from build123d import *

# Parameters (mm, degrees)
SKETCH1_R           = 22.225
SKETCH1_R_2         = 17.78
BOSS_EXTRUDE1_DEPTH = 50.8
SKETCH2_R           = 47.625
SKETCH2_R_2         = 22.225
BOSS_EXTRUDE2_DEPTH = 6.35
SKETCH3_R           = 3.175
CUT_EXTRUDE1_DEPTH  = 85.361847123
CHAMFER1_SIZE       = 1.27
BOSS_EXTRUDE3_DEPTH = 1.5875
CIRPATTERN1_COUNT   = 8
CUT_EXTRUDE3_DEPTH  = 85.361847123


with BuildPart() as part:
    # Sketch1 → Boss-Extrude1 (new body)
    with BuildSketch(Plane.XY):
        Circle(SKETCH1_R)
        Circle(SKETCH1_R_2, mode=Mode.SUBTRACT)
    extrude(amount=BOSS_EXTRUDE1_DEPTH)



with BuildPart() as body_2:
    # Sketch2 → Boss-Extrude2 (new body)
    with BuildSketch(Plane.XY.offset(50.8)):
        Circle(SKETCH2_R)
        Circle(SKETCH2_R_2, mode=Mode.SUBTRACT)
    extrude(amount=-BOSS_EXTRUDE2_DEPTH)

    # Sketch3 → Cut-Extrude1 (cut, through all)
    with BuildSketch(Plane.XY.offset(50.8)):
        with Locations((-38.1, 0)):
            Circle(SKETCH3_R)
        with Locations((-26.940768363, 26.940768363)):
            Circle(SKETCH3_R)
        with Locations((0, 38.1)):
            Circle(SKETCH3_R)
        with Locations((26.940768363, 26.940768363)):
            Circle(SKETCH3_R)
        with Locations((38.1, 0)):
            Circle(SKETCH3_R)
        with Locations((26.940768363, -26.940768363)):
            Circle(SKETCH3_R)
        with Locations((0, -38.1)):
            Circle(SKETCH3_R)
        with Locations((-26.940768363, -26.940768363)):
            Circle(SKETCH3_R)
    extrude(amount=-CUT_EXTRUDE1_DEPTH, mode=Mode.SUBTRACT)

    # Chamfer1
    chamfer1_edges = [body_2.edges().sort_by_distance(p)[0] for p in [
        (-47.625, 0, 44.45),
    ]]
    chamfer(chamfer1_edges, length=CHAMFER1_SIZE)


with BuildPart() as part_1:
    add(part.part)

    add(body_2.part)  # Boss-Extrude3 merges body 2
    # Sketch4 → Boss-Extrude3 (add, symmetric)
    with BuildSketch(Plane(origin=(0, 0, 0), x_dir=(0, 0, -1), z_dir=(0.9238795325112865, -0.3826834323650906, 0))):
        Polygon((-44.45, 34.925), (0, 22.225), (0, 21.463), (-44.45, 21.463), align=None)
    boss_extrude3 = extrude(amount=BOSS_EXTRUDE3_DEPTH, both=True)

    # CirPattern1: Boss-Extrude3 ×8 about axis
    cirpattern1_axis = Axis((0, 0, 0), (0, 0, 1))
    for i in range(1, CIRPATTERN1_COUNT):
        add(boss_extrude3.rotate(cirpattern1_axis, i * 360 / CIRPATTERN1_COUNT))

    # Sketch6 → Cut-Extrude3 (cut, through all)
    with BuildSketch(Plane(origin=(0, 0, 0), x_dir=(-1, 0, 0), z_dir=(0, 0, -1))):
        with BuildLine():
            ThreePointArc((-7.572075345, -16.087015726), (-17.372275069, -3.785823414), (-13.579066648, 11.477689183))
            Line((-13.579066648, 11.477689183), (-14.54899998, 12.297524124))
            ThreePointArc((-14.54899998, 12.297524124), (-18.61315186, -4.056239373), (-8.112937869, -17.236088278))
            Line((-8.112937869, -17.236088278), (-7.572075345, -16.087015726))
        make_face()
        with BuildLine():
            ThreePointArc((-10.145726618, 14.601117471), (5.407518283, 16.937743239), (16.729503733, 6.020972085))
            Line((16.729503733, 6.020972085), (17.924468285, 6.45104152))
            ThreePointArc((17.924468285, 6.45104152), (5.793769589, 18.147582041), (-10.870421376, 15.644054433))
            Line((-10.870421376, 15.644054433), (-10.145726618, 14.601117471))
        make_face()
        with BuildLine():
            Line((18.983359245, 1.592033845), (17.717801962, 1.485898255))
            ThreePointArc((17.717801962, 1.485898255), (17.764443685, 0.743599728), (17.78, 0))
            ThreePointArc((17.78, 0), (11.404245451, -13.640805903), (-3.150437085, -17.498661268))
            Line((-3.150437085, -17.498661268), (-3.375468305, -18.748565644))
            ThreePointArc((-3.375468305, -18.748565644), (12.81938227, -14.091342669), (18.983359245, 1.592033845))
        make_face()
    extrude(amount=-CUT_EXTRUDE3_DEPTH, mode=Mode.SUBTRACT)


solid = part_1.part
The listing builds one solid part. Answer for the finished solid, in the listing's coordinates (mm). A direction names the side the tool comes from. Coordinates: 2 decimals unless noted, no trailing zeros. Order: outer loops, then holes, each group sorted by start corner. A loop starts at its lowest first (then second) coordinate and runs counter-clockwise, first axis right, second up. Notation, with made-up numbers: (74, 26) -> (103, 26) arc R28 ccw to (103, 63) -> close; hole circle Ø3 at (47.5, 40.25). An arc over 180 degrees is marked (long way). Answer in a Markdown table with one row per item. Add a question column.
Item 1: Each of these flat-tipped pins is pushed along its axis until it touches: P1, Ø6, axis at y = 29, z = 23, coming from the -X side; P2, Ø1.5, axis at y = 16, z = 19, coming from the -X side; P3, Ø2, axis at y = 11, z = 9, coming from the -X side; P4, Ø5, axis at x = 26.94, y = -26.94, coming from the +Z side (3 decimals). Where does it stop, or does it pass through?
Item 2: Find section A-A (x = 0). Write down the section's boundary in (y, z) (3 decimals), then the cut area to 3 significant figures.
Item 3: Find the intervals of material crossed by L1, parallel to Y at x = 0, z = 46.5 (3 decimals); L2, parallel to Y at x = -29.5, z = 48.5; L3, parallel to Z at x = -4, y = -22, in increasing order. Write a range as from..to.
Item 4: Which of the six approach directions +Z, -Z, +X, -X, +Y, -Y give full straight-line access (tool end or side, diameter ignored) to faces 5 (the face through (22.225, -0.1, 21.914)), 6 (the face through (15.64, -15.79, 21.91)), 7 (the face through (-17.365, 3.818, 25.044)), 8 (the face through (-24.445, -8.407, 31.792))?
Item 5: Determine the mould class of faces 1 (the face through (-18, 5, 0)), 2 (the face through (26.473, -10.99, 22.536)), 3 (the face through (34.93, 0.14, 47.67)), 4 (the face through (15.79, 15.64, 21.91)) for opening direction Y: +Y half, -Y half, draft (parallel to the pull), parting line (faces both ways), or undercut.
Result set:
| question | item | result |
|---|---|---|
| 1 | P1 | stops at x = -12.65 |
| 1 | P2 | stops at x = -16.17 |
| 1 | P3 | stops at x = -22.8 |
| 1 | P4 | passes through |
| 2 | outline | (-47.625, 45.72) -> (-46.355, 44.45) -> (-41.275, 44.45) -> (-41.275, 50.8) -> (-47.625, 50.8) -> close; (-34.925, 44.45) -> (-22.225, 44.45) -> (-22.225, 0) -> (-19.05, 0) -> (-19.05, 50.8) -> (-34.925, 50.8) -> close; (19.05, 0) -> (22.225, 0) -> (22.225, 44.45) -> (34.925, 44.45) -> (34.925, 50.8) -> (19.05, 50.8) -> close; (41.275, 44.45) -> (46.355, 44.45) -> (47.625, 45.72) -> (47.625, 50.8) -> (41.275, 50.8) -> close |
| 2 | area | 563 mm² |
| 3 | L1 | y = -47.625..-41.275, -34.925..-19.05, 19.05..34.925, 41.275..47.625 |
| 3 | L2 | y = -37.39..-28.82, -25.06..25.06, 28.82..37.39 |
| 3 | L3 | z = 44.45..50.8 |
| 4 | face 5 | -Z, +X |
| 4 | face 6 | -Z |
| 4 | face 7 | +Z, -Z |
| 4 | face 8 | -Z, -X |
| 5 | face 1 | draft |
| 5 | face 2 | -Y half |
| 5 | face 3 | undercut |
| 5 | face 4 | undercut |
